Can you work these out from the model? Positions are in its coordinate system, mm. Face numbers are marked on the shaded views. A direction names the side the tool comes from. Coordinates: 2 decimals unless noted, no trailing zeros. Order: outer loops, then holes, each group sorted by start corner. A loop starts at its lowest first (then second) coordinate and runs counter-clockwise, first axis right, second up. Notation, with made-up numbers: (68, 80) -> (110, 80) arc R23 cw to (110, 109) -> close; hole circle Ø9 at (74.25, -27). An arc over 180 degrees is marked (long way). Answer as a JSON object with one key per item and string values. Group by question number.
(1) I want a section at A-A, the plane x = 133.5. List the corners of the cut face in (y, z) for me, plus the area to 3 significant figures.
(2) I want a section at B-B, the plane z = 147.5. List the corners of the cut face in (x, y) for me.
(3) For pin 1 (6 mm diameter, centred on x = 38.5, z = 97, fed in from +Y); pin 2 (10 mm diameter, centred on x = 105, z = 28, fed in from +Y), each with a flat end and sliding along its axis, tell me the tip position at first contact or that it passes through.
(4) I need wall thicknesses on line 1 (Y direction, x = 57, z = 88); line 2 (Y direction, x = 226, z = 25). Which ranges of each line are inside material? Lowest first, please.
(5) Which directions (+Z, -Z, +X, -X, +Y, -Y) give clear straight access to the entire face, cutting with the end or side of a thin tool? Please do the marked faces 1 and 2.
from build123d import *

# Parameters (mm, degrees)
F1_DEPTH = 268


with BuildPart() as f1:
    # F0 (on Right) → F1 (new body)
    with BuildSketch(Plane.YZ):
        with BuildLine():
            ThreePointArc((32, 0), (9.372583, 9.372583), (0, 32))
            Line((0, 32), (0, 162))
            Line((0, 162), (-0.2, 162))
            Line((-0.2, 162), (-0.2, 32))
            ThreePointArc((-0.2, 32), (9.231162, 9.231162), (32, -0.2))
            Line((32, -0.2), (332, -0.2))
            Line((332, -0.2), (332, 0))
            Line((332, 0), (32, 0))
        make_face()
    extrude(amount=F1_DEPTH)


solid = f1.part
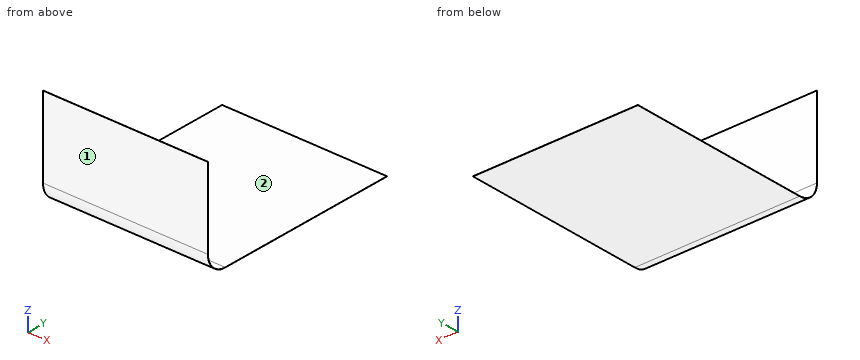
Computed values:
{
 "1": {"outline": "(-0.2, 32) arc R32.2 ccw to (32, -0.2) -> (332, -0.2) -> (332, 0) -> (32, 0) arc R32 cw to (0, 32) -> (0, 162) -> (-0.2, 162) -> close", "area": "96.1 mm2"},
 "2": {"outline": "(0, -0.2) -> (268, -0.2) -> (268, 0) -> (0, 0) -> close"},
 "3": {"pin 1": "stops at y = 0", "pin 2": "stops at y = 1.29"},
 "4": {"line 1": "y = -0.2 to 0", "line 2": "y = 0.57 to 0.78"},
 "5": {"face 1": "+Z, -Z, +X, -X, -Y", "face 2": "+Z, +X, -X, +Y"}
}
